Can you work these out from the drawing? Everything is in mm from the part's minimum corner. Coordinates: 2 decimals unless noted, no trailing zeros. Loops run counter-clockwise (first coordinate to the right, second up) from the corner with the lowest first, then second, coordinate; pieces in that order, holes last. Notation, with made-up numbers: (12, 3.5) -> (68, 3.5) arc R13 cw to (68, 25.5) -> close; hole circle Ø3 at (23, 74). An arc over 180 degrees is marked (long way). One line per question, with ' | ' between items.
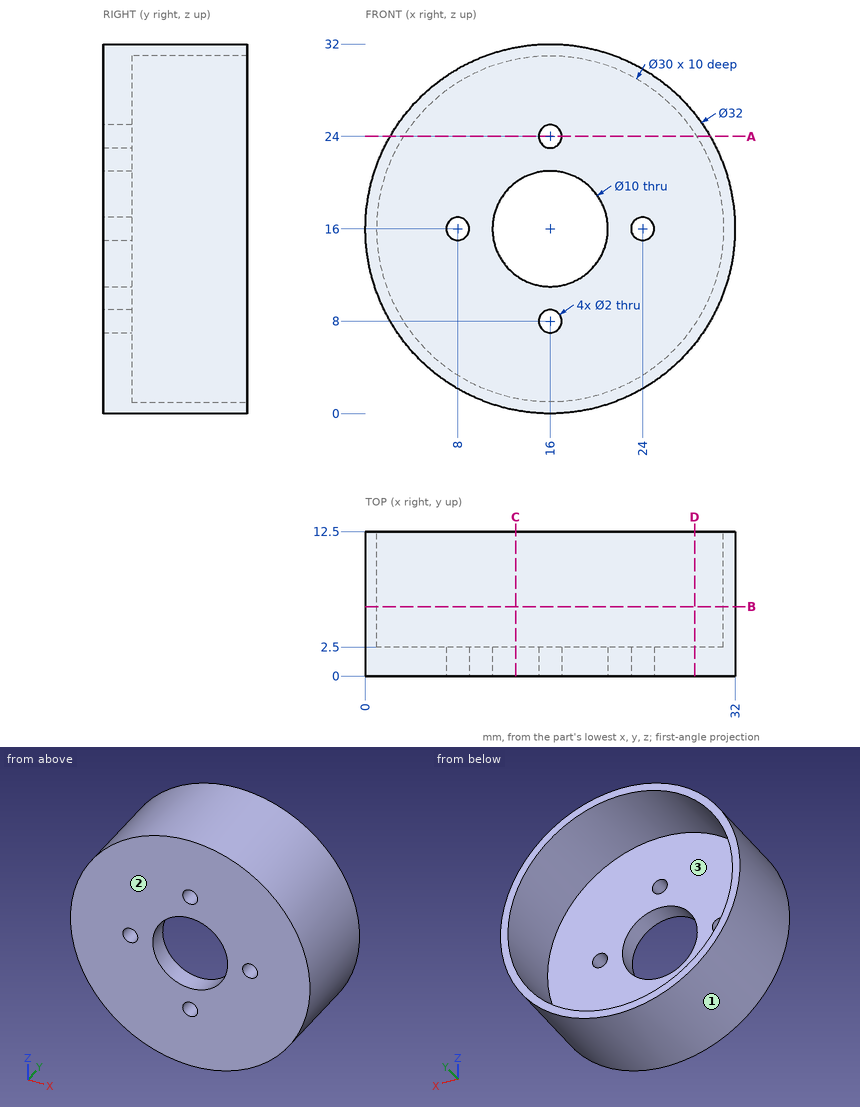
Q1. We'd pull the mould along Z, two halves only. Please class the marked faces 1, 2 and 3: released by +Z, released by -Z, zero draft, split by the parting line, or undercut.
Values follow:
face 1: split by the parting line | face 2: zero draft | face 3: undercut
Q2. Please list where these lines run through material, in increasing order: L1, parallel to X at y = 1.75, z = 16; L2, parallel to Y at x = 15.5, z = 22.5; L3, parallel to Z at x = 5.5, y = 10.75. Write a range as [from, to].
Values follow:
L1: x = [0, 7], [9, 11], [21, 23], [25, 32] | L2: y = [0, 2.5] | L3: z = [3.93, 5.29], [26.71, 28.07]
Q3. Imagine slicing it at D-D on x = 28.5. Write out the boundary of the cut face in (y, z), plus the area to 3 significant figures.
Values follow:
outline: (0, 6.01) -> (12.5, 6.01) -> (12.5, 7.71) -> (2.5, 7.71) -> (2.5, 24.29) -> (12.5, 24.29) -> (12.5, 25.99) -> (0, 25.99) -> close | area: 83.9 mm2
Q4. Imagine slicing it at B-B on y = 6. Write out the boundary of the cut face in (x, z).
Values follow:
outline: circle Ø32 at (16, 16); hole circle Ø30 at (16, 16)
Q5. For pin 1 (6 mm diameter, centred on x = 6.5, z = 10, fed in from +Y); pin 2 (5 mm diameter, centred on y = 7.5, z = 4, fed in from -X); pin 3 (6 mm diameter, centred on y = 4, z = 8, fed in from +X), each with a flat end and sliding along its axis, tell me the tip position at first contact or that it passes through.
Values follow:
pin 1: stops at y = 2.5 | pin 2: stops at x = 3.13 | pin 3: stops at x = 31.2
Q6. Imagine slicing it at C-C on x = 13. Write out the boundary of the cut face in (y, z).
Values follow:
outline: (0, 0.28) -> (12.5, 0.28) -> (12.5, 1.3) -> (2.5, 1.3) -> (2.5, 12) -> (0, 12) -> close; (0, 20) -> (2.5, 20) -> (2.5, 30.7) -> (12.5, 30.7) -> (12.5, 31.72) -> (0, 31.72) -> close
Q7. Imagine slicing it at A-A on z = 24. Write out the boundary of the cut face in (x, y), plus the area to 3 significant figures.
Values follow:
outline: (2.14, 0) -> (15, 0) -> (15, 2.5) -> (3.31, 2.5) -> (3.31, 12.5) -> (2.14, 12.5) -> close; (17, 0) -> (29.86, 0) -> (29.86, 12.5) -> (28.69, 12.5) -> (28.69, 2.5) -> (17, 2.5) -> close | area: 87.6 mm2
